CAD build for the part. Positions are in the model's coordinates, mm. Face numbers are marked on the shaded views. A direction names the side the tool comes from. Give positions to 0.01 mm unless a question says otherwise; leave off trailing zeros. Write each loop counter-clockwise with the first axis right and the second up, starting at its lowest first coordinate (ties: lowest second). Pieces come first, ordered by that corner, then holes. Notation, with made-up numbers: (-25, -5) - (-7, -5) arc R28 cw to (-7, 34) - close; hole circle Ø7 at (-32.5, -19.75). An arc over 180 degrees is marked (long way). Answer as a JSON object with one key per item and string values.
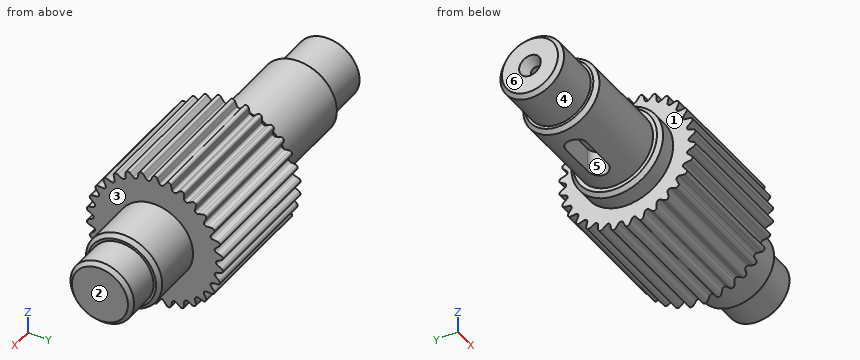
from build123d import *

# Parameters (mm, degrees)
CUT_EXTRUDE_START        = -10
CUT_EXTRUDE_1_DEPTH      = 168.009171707
CUT_EXTRUDE_3_REACH      = 121.806
PATTERN_CIRCULAR_4_COUNT = 30
FILLET_4_R               = 1
CHAMFER_1_SIZE           = 1.5


with BuildPart() as part:
    # Эскиз1 → Повернуть1 (revolve)
    with BuildSketch(Plane.XY, mode=Mode.PRIVATE) as revolve_1_sk:
        Polygon((54.670592349, -18), (62.670592349, -18), (62.670592349, -28.8), (112.670592349, -28.8), (112.670592349, -15), (134, -15), (134, -12.5), (148, -12.5), (148, 0), (0, 0), (0, -12.5), (18.670592349, -12.5), (18.670592349, -15), (54.670592349, -15), align=None)
    revolve(revolve_1_sk.sketch.rotate(Axis((0, 0, 0), (1, 0, 0)), 270), axis=Axis((0, 0, 0), (1, 0, 0)))

    # Эскиз2 → Вырез-Повернуть1 (revolve, cut)
    with BuildSketch(Plane.XY, mode=Mode.PRIVATE) as cut_revolve_1_sk:
        Polygon((0, 0), (0, 4.25), (3.9, 2), (8.9, 2), (10.054700538, 0), align=None)
    revolve(cut_revolve_1_sk.sketch.rotate(Axis((0, 0, 0), (1, 0, 0)), 90), axis=Axis((0, 0, 0), (1, 0, 0)), mode=Mode.SUBTRACT)

    # Эскиз3 → Вырез-Вытянуть1 (cut, through all)
    with BuildSketch(Plane(origin=(0, 0, -15), x_dir=(-1, 0, 0), z_dir=(0, 0, -1)).offset(CUT_EXTRUDE_START)):
        with BuildLine():
            Line((-29.670592349, -4), (-43.670592349, -4))
            ThreePointArc((-43.670592349, -4), (-47.670592349, 0), (-43.670592349, 4))
            Line((-43.670592349, 4), (-29.670592349, 4))
            ThreePointArc((-29.670592349, 4), (-25.670592349, 0), (-29.670592349, -4))
        make_face()
    extrude(amount=CUT_EXTRUDE_1_DEPTH, mode=Mode.SUBTRACT)

    # Эскиз4 → Вырез-Вытянуть3 (cut, up to next)
    with BuildSketch(Plane(origin=(112.670592349, 0, 0), x_dir=(0, 0, -1), z_dir=(1, 0, 0)), mode=Mode.PRIVATE) as cut_extrude_3_sk1:
        Polygon((5, 31.686751346), (-5, 31.686751346), (0, 23.026497308), align=None)
    cut_extrude_3_tool1 = extrude(cut_extrude_3_sk1.sketch, amount=-CUT_EXTRUDE_3_REACH, mode=Mode.PRIVATE) & part.part
    cut_extrude_3 = cut_extrude_3_tool1.solids().sort_by_distance((112.670592, 28.8, 0))[0]
    add(cut_extrude_3, mode=Mode.SUBTRACT)

    # Круговой массив4: Вырез-Вытянуть3 ×30 about axis
    pattern_circular_4_axis = Axis((0, 0, 0), (1, 0, 0))
    for i in range(1, PATTERN_CIRCULAR_4_COUNT):
        add(cut_extrude_3.rotate(pattern_circular_4_axis, i * 360 / PATTERN_CIRCULAR_4_COUNT), mode=Mode.SUBTRACT)

    # Скругление4
    fillet_4_edges = [part.edges().sort_by_distance(p)[0] for p in [
        (87.670592349, 28.15133101, -2.958824118),
        (87.670592349, 22.523313095, -4.787477989),
        (87.670592349, 26.92098276, -8.747157541),
        (87.670592349, 21.035752021, -9.365720217),
        (87.670592349, 24.514058382, -14.153198206),
        (87.670592349, 18.628827643, -13.53463553),
        (87.670592349, 21.035752021, -18.940676195),
        (87.670592349, 15.407734106, -17.112022323),
        (87.670592349, 16.638082356, -22.900355747),
        (87.670592349, 11.513248654, -19.941531629),
        (87.670592349, 11.513248654, -25.859179864),
        (87.670592349, 7.115578989, -21.899500312),
        (87.670592349, 5.885230739, -27.687833735),
        (87.670592349, 2.406924378, -22.900355747),
        (87.670592349, 0, -28.306396412),
        (87.670592349, -2.406924378, -22.900355747),
        (87.670592349, -5.885230739, -27.687833735),
        (87.670592349, -7.115578989, -21.899500312),
        (87.670592349, -11.513248654, -25.859179864),
        (87.670592349, -11.513248654, -19.941531629),
        (87.670592349, -16.638082356, -22.900355747),
        (87.670592349, -15.407734106, -17.112022323),
        (87.670592349, -21.035752021, -18.940676195),
        (87.670592349, -18.628827643, -13.53463553),
        (87.670592349, -24.514058382, -14.153198206),
        (87.670592349, -21.035752021, -9.365720217),
        (87.670592349, -26.92098276, -8.747157541),
        (87.670592349, -22.523313095, -4.787477989),
        (87.670592349, -28.15133101, -2.958824118),
        (87.670592349, -23.026497308, 0),
        (87.670592349, -28.15133101, 2.958824118),
        (87.670592349, -22.523313095, 4.787477989),
        (87.670592349, -26.92098276, 8.747157541),
        (87.670592349, -21.035752021, 9.365720217),
        (87.670592349, -24.514058382, 14.153198206),
        (87.670592349, -18.628827643, 13.53463553),
        (87.670592349, -21.035752021, 18.940676195),
        (87.670592349, -15.407734106, 17.112022323),
        (87.670592349, -16.638082356, 22.900355747),
        (87.670592349, -11.513248654, 19.941531629),
        (87.670592349, -11.513248654, 25.859179864),
        (87.670592349, -7.115578989, 21.899500312),
        (87.670592349, -5.885230739, 27.687833735),
        (87.670592349, -2.406924378, 22.900355747),
        (87.670592349, 0, 28.306396412),
        (87.670592349, 2.406924378, 22.900355747),
        (87.670592349, 5.885230739, 27.687833735),
        (87.670592349, 7.115578989, 21.899500312),
        (87.670592349, 11.513248654, 25.859179864),
        (87.670592349, 11.513248654, 19.941531629),
        (87.670592349, 16.638082356, 22.900355747),
        (87.670592349, 15.407734106, 17.112022323),
        (87.670592349, 21.035752021, 18.940676195),
        (87.670592349, 18.628827643, 13.53463553),
        (87.670592349, 24.514058382, 14.153198206),
        (87.670592349, 21.035752021, 9.365720217),
        (87.670592349, 28.15133101, 2.958824118),
        (87.670592349, 26.92098276, 8.747157541),
        (87.670592349, 22.523313095, 4.787477989),
        (87.670592349, 23.026497308, 0),
    ]]
    fillet(fillet_4_edges, radius=FILLET_4_R)

    # Фаска1
    chamfer_1_edges = [part.edges().sort_by_distance(p)[0] for p in [
        (54.670592349, 0, -18),
        (18.670592349, 0, -15),
        (0, 0, -12.5),
        (148, 0, -12.5),
        (134, 0, -15),
    ]]
    chamfer(chamfer_1_edges, length=CHAMFER_1_SIZE)


solid = part.part
(1) Saw through at A-A, the plane x = 37. Give the cut face in (y, z), and give its area (3 significant figures).
Answer key:
{"outline": "(-4, -14.46) - (-4, -5) - (4, -5) - (4, -14.46) arc R15 ccw (long way) to start", "area": "628 mm²"}
(2) Probe L1, parallel to Y at x = 6.9, z = 0; L2, parallel to Z at x = 111, y = 23; L3, parallel to Z at x = 13, y = 0.5. List the from-to ranges inside material, lowest first. Write a range as [from, to].
Answer key:
{"L1": "y = [-12.5, -2], [2, 12.5]", "L2": "z = [-13.71, -12.07], [-9.16, 9.16], [12.07, 13.71]", "L3": "z = [-12.49, 12.49]"}
(3) Saw through at B-B, the plane x = 122. Give the cut face in (y, z), and give its area (3 significant figures).
Answer key:
{"outline": "circle Ø30 at (0, 0)", "area": "707 mm²"}
(4) Pull direction Y, two halves, no side cores. Call the marked faces 4, 5 and 6: pulls with the +Y half, pulls with the -Y half, needs draft (parallel to the pull), parting line crosses it, or undercut.
Answer key:
{"face 4": "parting line crosses it", "face 5": "undercut", "face 6": "needs draft"}
(5) 3-axis set-ups, long thin cutter, end or side, ignore diameter. For the marked faces 1, 2 and 3: which of +Z, -Z, +X, -X, +Y, -Y reach the whole face in a straight line?
Answer key:
{"face 1": "-X", "face 2": "+Z, -Z, +X, +Y, -Y", "face 3": "+X"}
(6) Flat gauge pins, fed straight in: P1, Ø4.5, axis at x = 34.5, z = -11, coming from the +Y side; P2, Ø1, axis at x = 97, z = -23, coming from the +Y side; P3, Ø10, axis at x = 98.5, z = 12.5, coming from the -Y side. Where does each tip first touch, or does it go through?
Answer key:
{"P1": "stops at y = 12.18", "P2": "stops at y = 11.51", "P3": "stops at y = -25.58"}
